```python
from build123d import *

# Parameters (mm, degrees)
F0_W     = 203.2
F0_H     = 50.8
F1_DEPTH = 25.4
F2_W     = 19.05
F2_H     = 44.45
F3_DEPTH = 304.8
F5_DEPTH = 25.4


with BuildPart() as f1:
    # F0 (on Front) → F1 (new body)
    with BuildSketch(Plane.XZ):
        with Locations((101.6, 25.4)):
            Rectangle(F0_W, F0_H)
    extrude(amount=F1_DEPTH)

    # F2 (on face) → F3 (cut)
    with BuildSketch(Plane(origin=(0, 0, 0), x_dir=(0, -1, 0), z_dir=(-1, 0, 0))):
        with Locations((12.7, 25.4)):
            Rectangle(F2_W, F2_H)
    extrude(amount=-F3_DEPTH, mode=Mode.SUBTRACT)

    # F4 (on face) → F5 (cut)
    with BuildSketch(Plane.XZ.offset(25.4)):
        Polygon((54.466174, 31.75), (47.133826, 31.75), (43.467652, 25.4), (47.133826, 19.05), (54.466174, 19.05), (58.132348, 25.4), align=None)
    extrude(amount=-F5_DEPTH, mode=Mode.SUBTRACT)


solid = f1.part
```
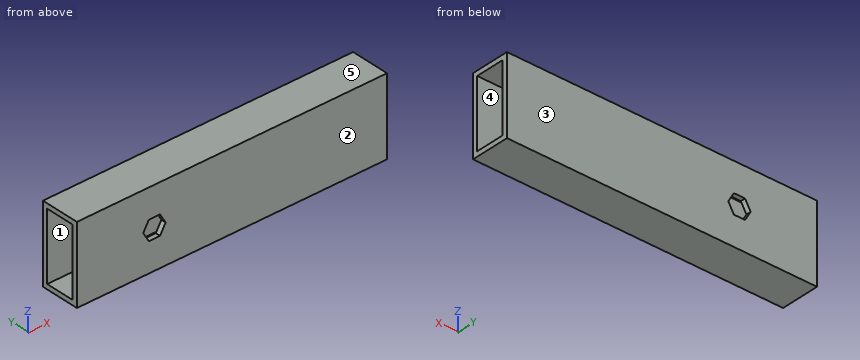
Work out the finished part from the listing and answer in its coordinate system (mm). Face numbers are marked on the shaded views. A direction names the side the tool comes from. Coordinates: 2 decimals unless noted, no trailing zeros. Write each loop counter-clockwise with the first axis right and the second up, starting at its lowest first coordinate (ties: lowest second). Pieces come first, ordered by that corner, then holes.
Q1. Which of the six approach directions +Z, -Z, +X, -X, +Y, -Y give full straight-line access (tool end or side, diameter ignored) to the marked faces 1 and 2?
Q2. A cutting plane is placed at D-D, the plane z = 28.5. Give the vertices of the cut face in (x, y) (3 decimals).
Q3. Find the intervals of material crossed by line 1 (Y direction, x = 71, z = 47) (3 decimals); line 2 (Z direction, x = 60, y = -19) (3 decimals), in increasing order.
Q4. A cutting plane is placed at B-B, the plane x = 150. Give the vertices of the cut face in (y, z) (3 decimals), then the cut area to 3 significant figures.
Q5. Determine the mould class of the marked faces 3, 4 and 5 for opening direction Z: released by +Z, released by -Z, zero draft, split by the parting line, or undercut.
Q6. A cutting plane is placed at C-C, the plane y = -12.5. Give the vertices of the cut face in (x, z) (3 decimals), then the cut area to 3 significant figures.
Q7. A cutting plane is placed at A-A, the plane z = 40. Give the vertices of the cut face in (x, y) (3 decimals), then the cut area to 3 significant figures.
Findings below:
1. face 1: +X, -X
1. face 2: +Z, -Z, +X, -X, -Y
2. outline: (0, -25.4) - (45.257, -25.4) - (45.257, -22.225) - (0, -22.225) - close; (0, -3.175) - (45.257, -3.175) - (45.257, 0) - (0, 0) - close; (56.343, -25.4) - (203.2, -25.4) - (203.2, -22.225) - (56.343, -22.225) - close; (56.343, -3.175) - (203.2, -3.175) - (203.2, 0) - (56.343, 0) - close
3. line 1: y = -25.4 to -22.225, -3.175 to 0
3. line 2: z = 0 to 3.175, 47.625 to 50.8
4. outline: (-25.4, 0) - (0, 0) - (0, 50.8) - (-25.4, 50.8) - close; hole (-22.225, 3.175) - (-3.175, 3.175) - (-3.175, 47.625) - (-22.225, 47.625) - close
4. area: 444 mm2
5. face 3: zero draft
5. face 4: undercut
5. face 5: released by +Z
6. outline: (0, 0) - (203.2, 0) - (203.2, 3.175) - (0, 3.175) - close; (0, 47.625) - (203.2, 47.625) - (203.2, 50.8) - (0, 50.8) - close
6. area: 1,290 mm2
7. outline: (0, -25.4) - (203.2, -25.4) - (203.2, -22.225) - (0, -22.225) - close; (0, -3.175) - (203.2, -3.175) - (203.2, 0) - (0, 0) - close
7. area: 1,290 mm2
